For this review, take the finished solid that the model builds, in its own axes (mm). Face numbers are marked on the shaded views. A direction names the side the tool comes from. Round coordinates to 2 decimals unless told otherwise and drop trailing zeros. Order: outer loops, then holes, each group sorted by start corner. A loop starts at its lowest first (then second) coordinate and runs counter-clockwise, first axis right, second up. Notation, with made-up numbers: M 87,71 L 94,71 A19 ccw 94,81 Z; hole C 85.25,69 d3. An arc over 180 degrees is marked long. Use a Markdown table: item, result.
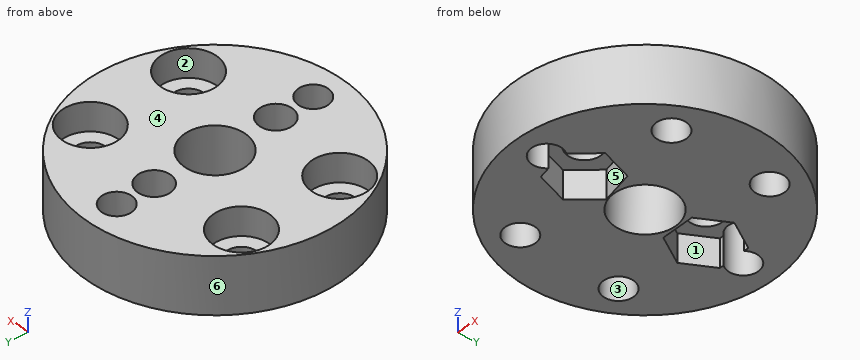
from build123d import *

# Parameters (mm, degrees)
SKETCH_1_R          = 13.75
SKETCH_1_R_2        = 1.6
SKETCH_1_R_3        = 3.25
EXTRUDE_1_DEPTH     = 6
SKETCH_2_R          = 1.75
CUT_EXTRUDE_1_DEPTH = 7
SKETCH_3_R          = 3
CUT_EXTRUDE_2_DEPTH = 3
CUT_EXTRUDE_6_DEPTH = 3


with BuildPart() as part:
    # ｽｹｯﾁ1 → ﾎﾞｽ - 押し出し1 (new body)
    with BuildSketch(Plane.XY):
        Circle(SKETCH_1_R)
        with Locations((0, 10.5)):
            Circle(SKETCH_1_R_2, mode=Mode.SUBTRACT)
        with Locations((9.09326674, 5.25)):
            Circle(SKETCH_1_R_2, mode=Mode.SUBTRACT)
        with Locations((9.09326674, -5.25)):
            Circle(SKETCH_1_R_2, mode=Mode.SUBTRACT)
        with Locations((0, -10.5)):
            Circle(SKETCH_1_R_2, mode=Mode.SUBTRACT)
        with Locations((-9.09326674, -5.25)):
            Circle(SKETCH_1_R_2, mode=Mode.SUBTRACT)
        with Locations((-9.09326674, 5.25)):
            Circle(SKETCH_1_R_2, mode=Mode.SUBTRACT)
        Circle(SKETCH_1_R_3, mode=Mode.SUBTRACT)
    extrude(amount=EXTRUDE_1_DEPTH)

    # ｽｹｯﾁ2 → ｶｯﾄ - 押し出し1 (cut, through all)
    with BuildSketch(Plane.XY.offset(6)):
        with Locations((0, 6.5)):
            Circle(SKETCH_2_R)
        with Locations((0, -6.5)):
            Circle(SKETCH_2_R)
    extrude(amount=-CUT_EXTRUDE_1_DEPTH, mode=Mode.SUBTRACT)

    # ｽｹｯﾁ3 → ｶｯﾄ - 押し出し2 (cut)
    with BuildSketch(Plane.XY.offset(6)):
        with Locations((9.09326674, 5.25)):
            Circle(SKETCH_3_R)
        with Locations((-9.09326674, -5.25)):
            Circle(SKETCH_3_R)
        with Locations((-9.09326674, 5.25)):
            Circle(SKETCH_3_R)
        with Locations((9.09326674, -5.25)):
            Circle(SKETCH_3_R)
    extrude(amount=-CUT_EXTRUDE_2_DEPTH, mode=Mode.SUBTRACT)

    # ｽｹｯﾁ7 → ｶｯﾄ - 押し出し6 (cut)
    with BuildSketch(Plane(origin=(0, 0, 0), x_dir=(-1, 0, 0), z_dir=(0, 0, -1))):
        Polygon((1.752709389, 3.512022457), (3.464019153, 6.523902085), (1.711309763, 9.511879628), (-1.752709389, 9.487977543), (-3.464019153, 6.476097915), (-1.711309763, 3.488120372), align=None)
        Polygon((2.335754412, -9.058173436), (3.383320389, -5.75626406), (1.047565977, -3.198090624), (-2.335754412, -3.941826564), (-3.383320389, -7.24373594), (-1.047565977, -9.801909376), align=None)
    extrude(amount=-CUT_EXTRUDE_6_DEPTH, mode=Mode.SUBTRACT)


solid = part.part
Q1. Add section C-C (z = 3.7). Give the number of separate pieces and of enclosed holes in the cut face, then the cut area to 3 significant figures.
Determined:
| item | result |
|---|---|
| separate pieces | 1 |
| enclosed holes | 9 |
| area | 412 mm^2 |
Q2. Draft analysis for pull direction Y (two halves, no side actions). For the marked faces 4, 5 and 6, state which applies: pulls with the +Y half, pulls with the -Y half, needs draft (parallel to the pull), parting line crosses it, or undercut.
Determined:
| item | result |
|---|---|
| face 4 | needs draft |
| face 5 | undercut |
| face 6 | parting line crosses it |
Q3. Clearance check with flat-ended pins moving along their axes: pin 1 (7 mm diameter, centred on x = 9.09, y = 5.25, fed in from -Z); pin 2 (3 mm diameter, centred on x = 0, y = 6.5, fed in from -Z); pin 3 (1.9 mm diameter, centred on x = -1, y = -5, fed in from -Z); pin 4 (3.5 mm diameter, centred on x = -9.09, y = 5.25, fed in from +Z). State where each tip first meets the part, or that it passes through.
Determined:
| item | result |
|---|---|
| pin 1 | stops at z = 0 |
| pin 2 | passes through |
| pin 3 | stops at z = 3 |
| pin 4 | stops at z = 3 |
Q4. Machinability: for the marked faces 1, 2 and 3, which of the approach directions +Z, -Z, +X, -X, +Y, -Y give a long, thin tool a straight path to every point of the face, cutting with its end or side? Answer none if there is none.
Determined:
| item | result |
|---|---|
| face 1 | -Z |
| face 2 | +Z |
| face 3 | +Z, -Z |
Q5. Add section B-B (z = 1.1). Write out the cut boundary in (x, y), then the cut area to 3 significant figures.
Determined:
| item | result |
|---|---|
| outline | C 0,0 d27.5; hole C -9.09,-5.25 d3.2; hole C -9.09,5.25 d3.2; hole M -3.46,6.52 L -1.75,3.51 L 1.71,3.49 L 3.46,6.48 L 1.75,9.49 L 1.24,9.49 A1.6 ccw long -1.26,9.51 L -1.71,9.51 Z; hole M -3.38,-5.76 L -2.34,-9.06 L -1.09,-9.33 A1.6 ccw long 1.28,-9.54 L 3.38,-7.24 L 2.34,-3.94 L -1.05,-3.2 Z; hole C 0,0 d6.5; hole C 9.09,-5.25 d3.2; hole C 9.09,5.25 d3.2 |
| area | 452 mm^2 |
Q6. Add section D-D (x = 0). Write out the cut boundary in (y, z).
Determined:
| item | result |
|---|---|
| outline | M -13.75,0 L -12.1,0 L -12.1,6 L -13.75,6 Z; M -8.9,3 L -8.25,3 L -8.25,6 L -8.9,6 Z; M -4.75,3 L -3.43,3 L -3.43,0 L -3.25,0 L -3.25,6 L -4.75,6 Z; M 3.25,0 L 3.5,0 L 3.5,3 L 4.75,3 L 4.75,6 L 3.25,6 Z; M 8.25,3 L 8.9,3 L 8.9,6 L 8.25,6 Z; M 12.1,0 L 13.75,0 L 13.75,6 L 12.1,6 Z |
Q7. Add section A-A (y = 0). Write out the cut boundary in (x, z), then the cut area to 3 significant figures.
Determined:
| item | result |
|---|---|
| outline | M -13.75,0 L -3.25,0 L -3.25,6 L -13.75,6 Z; M 3.25,0 L 13.75,0 L 13.75,6 L 3.25,6 Z |
| area | 126 mm^2 |
Q8. Wall thickness on line 1 along Y through (x, z) = (0, 4.7); line 2 along Y through (x, z) = (10, 1.9); line 3 along Y through (x, z) = (-11.75, 4.9): over which ranges is each line inside the solid? List them lowest first. Write a range as [from, to].
Determined:
| item | result |
|---|---|
| line 1 | y = [-13.75, -12.1], [-8.9, -8.25], [-4.75, -3.25], [3.25, 4.75], [8.25, 8.9], [12.1, 13.75] |
| line 2 | y = [-9.44, -6.57], [-3.93, 3.93], [6.57, 9.44] |
| line 3 | y = [-7.14, -6.64], [-3.86, 3.86], [6.64, 7.14] |
